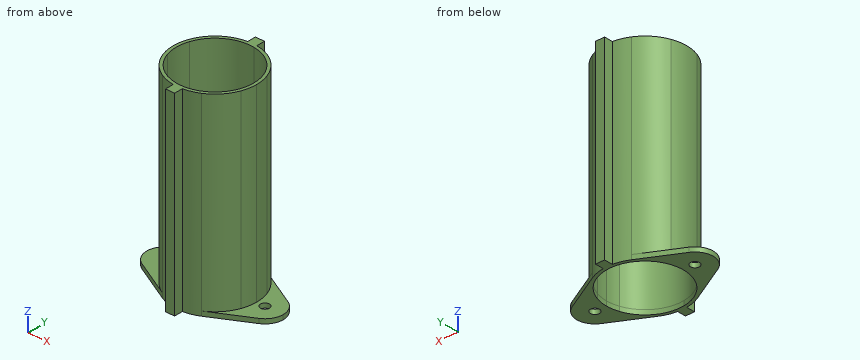
```python
from build123d import *
from build123d import SkipClean  # not in build123d's __all__

# Parameters (mm, degrees)
F0_R     = 3
F1_DEPTH = 3
F2_DEPTH = 125


# Not quite as in the source:
# - a feature names something its author has since deleted; it is built from what else it names


with BuildPart() as f1:
    # F0 (on Top) → F1 (new body)
    with BuildSketch(Plane.XY):
        with BuildLine():
            ThreePointArc((12.9166666896, 24.2777618744), (20.6949130465, 18.1099578685), (25.7765151515, 9.5823413967))
            ThreePointArc((25.7765151515, 9.5823413967), (32.0589540907, 11.9630444535), (38.6363637791, 10.5939323837))
            Line((38.6363637791, 10.5939323837), (12.9166666896, 24.2777618744))
        make_face()
        with BuildLine():
            ThreePointArc((25.7765151515, 9.5823413967), (27.0656993875, 4.8680506023), (27.5, 0))
            ThreePointArc((27.5, 0), (27.0656993875, -4.8680506023), (25.7765151515, -9.5823413967))
            ThreePointArc((25.7765151515, -9.5823413967), (32.0589541175, -11.9630444556), (38.6363638266, -10.5939323584))
            ThreePointArc((38.6363638266, -10.5939323584), (43.2867965353, -6.1791437142), (45, 0))
            ThreePointArc((45, 0), (43.2867965215, 6.1791437372), (38.6363637791, 10.5939323837))
            ThreePointArc((38.6363637791, 10.5939323837), (32.0589540907, 11.9630444535), (25.7765151515, 9.5823413967))
        make_face()
        with Locations((33, 0)):
            Circle(F0_R, mode=Mode.SUBTRACT)
        with BuildLine():
            ThreePointArc((25.7765151515, -9.5823413967), (27.0656993875, -4.8680506023), (27.5, 0))
            ThreePointArc((27.5, 0), (27.0656993875, 4.8680506023), (25.7765151515, 9.5823413967))
            ThreePointArc((25.7765151515, 9.5823413967), (24.9405426226, 8.8907337595), (24.1704545455, 8.1264461523))
            ThreePointArc((24.1704545455, 8.1264461523), (25.1654186425, 4.117244776), (25.5, 0))
            ThreePointArc((25.5, 0), (25.1654186425, -4.117244776), (24.1704545455, -8.1264461523))
            ThreePointArc((24.1704545455, -8.1264461523), (24.9405426226, -8.8907337595), (25.7765151515, -9.5823413967))
        make_face()
        with BuildLine():
            ThreePointArc((-3, 27.3358738657), (0, 27.5), (3, 27.3358738657))
            Line((3, 27.3358738657), (3, 33))
            Line((3, 33), (-3, 33))
            Line((-3, 33), (-3, 27.3358738657))
        make_face()
        with BuildLine():
            ThreePointArc((38.6363638266, -10.5939323584), (32.0589541175, -11.9630444556), (25.7765151515, -9.5823413967))
            ThreePointArc((25.7765151515, -9.5823413967), (20.6949131964, -18.1099576972), (12.9166670915, -24.2777616606))
            Line((12.9166670915, -24.2777616606), (38.6363638266, -10.5939323584))
        make_face()
        with BuildLine():
            ThreePointArc((-25.7765151515, 9.5823413967), (-20.6949129227, 18.1099580099), (-12.9166663578, 24.2777620509))
            Line((-12.9166663578, 24.2777620509), (-38.636363452, 10.5939325577))
            ThreePointArc((-38.636363452, 10.5939325577), (-32.058953906, 11.963044439), (-25.7765151515, 9.5823413967))
        make_face()
        with BuildLine():
            ThreePointArc((-25.7765151515, -9.5823413967), (-27.5, 0), (-25.7765151515, 9.5823413967))
            ThreePointArc((-25.7765151515, 9.5823413967), (-32.058953906, 11.963044439), (-38.636363452, 10.5939325577))
            ThreePointArc((-38.636363452, 10.5939325577), (-45, 1.496e-07), (-38.6363637162, -10.5939324171))
            ThreePointArc((-38.6363637162, -10.5939324171), (-32.0589540552, -11.9630444507), (-25.7765151515, -9.5823413967))
        make_face()
        with Locations((-33, 0)):
            Circle(F0_R, mode=Mode.SUBTRACT)
        with BuildLine():
            ThreePointArc((-24.1704545455, -8.1264461523), (-25.5, 0), (-24.1704545455, 8.1264461523))
            ThreePointArc((-24.1704545455, 8.1264461523), (-24.9405426226, 8.8907337595), (-25.7765151515, 9.5823413967))
            ThreePointArc((-25.7765151515, 9.5823413967), (-27.5, 0), (-25.7765151515, -9.5823413967))
            ThreePointArc((-25.7765151515, -9.5823413967), (-24.9405426226, -8.8907337595), (-24.1704545455, -8.1264461523))
        make_face()
        with BuildLine():
            Line((-38.6363637162, -10.5939324171), (-12.9166665881, -24.2777619284))
            ThreePointArc((-12.9166665881, -24.2777619284), (-20.6949130086, -18.1099579118), (-25.7765151515, -9.5823413967))
            ThreePointArc((-25.7765151515, -9.5823413967), (-32.0589540552, -11.9630444507), (-38.6363637162, -10.5939324171))
        make_face()
        with BuildLine():
            Line((3, 25.3229145242), (3, 27.3358738657))
            ThreePointArc((3, 27.3358738657), (0, 27.5), (-3, 27.3358738657))
            Line((-3, 27.3358738657), (-3, 25.3229145242))
            ThreePointArc((-3, 25.3229145242), (0, 25.5), (3, 25.3229145242))
        make_face()
        with BuildLine():
            ThreePointArc((24.1704545455, 8.1264461523), (24.9405426226, 8.8907337595), (25.7765151515, 9.5823413967))
            ThreePointArc((25.7765151515, 9.5823413967), (20.6949130465, 18.1099578685), (12.9166666896, 24.2777618744))
            ThreePointArc((12.9166666896, 24.2777618744), (8.1038930067, 26.2788302277), (3, 27.3358738657))
            Line((3, 27.3358738657), (3, 25.3229145242))
            ThreePointArc((3, 25.3229145242), (16.0775629735, 19.7929777657), (24.1704545455, 8.1264461523))
        make_face()
        with BuildLine():
            Line((-3, 25.3229145242), (-3, 27.3358738657))
            ThreePointArc((-3, 27.3358738657), (-8.1038928272, 26.2788302831), (-12.9166663578, 24.2777620509))
            ThreePointArc((-12.9166663578, 24.2777620509), (-20.6949129227, 18.1099580099), (-25.7765151515, 9.5823413967))
            ThreePointArc((-25.7765151515, 9.5823413967), (-24.9405426226, 8.8907337595), (-24.1704545455, 8.1264461523))
            ThreePointArc((-24.1704545455, 8.1264461523), (-16.0775629735, 19.7929777657), (-3, 25.3229145242))
        make_face()
        with BuildLine():
            ThreePointArc((-3, -27.3358738657), (0, -27.5), (3, -27.3358738657))
            Line((3, -27.3358738657), (3, -25.3229145242))
            ThreePointArc((3, -25.3229145242), (0, -25.5), (-3, -25.3229145242))
            Line((-3, -25.3229145242), (-3, -27.3358738657))
        make_face()
        with BuildLine():
            Line((3, -33), (3, -27.3358738657))
            ThreePointArc((3, -27.3358738657), (0, -27.5), (-3, -27.3358738657))
            Line((-3, -27.3358738657), (-3, -33))
            Line((-3, -33), (3, -33))
        make_face()
        with BuildLine():
            ThreePointArc((12.9166670915, -24.2777616606), (20.6949131964, -18.1099576972), (25.7765151515, -9.5823413967))
            ThreePointArc((25.7765151515, -9.5823413967), (24.9405426226, -8.8907337595), (24.1704545455, -8.1264461523))
            ThreePointArc((24.1704545455, -8.1264461523), (16.0775629735, -19.7929777657), (3, -25.3229145242))
            Line((3, -25.3229145242), (3, -27.3358738657))
            ThreePointArc((3, -27.3358738657), (8.1038932243, -26.2788301606), (12.9166670915, -24.2777616606))
        make_face()
        with BuildLine():
            ThreePointArc((-12.9166665881, -24.2777619284), (-8.1038929518, -26.2788302446), (-3, -27.3358738657))
            Line((-3, -27.3358738657), (-3, -25.3229145242))
            ThreePointArc((-3, -25.3229145242), (-16.0775629735, -19.7929777657), (-24.1704545455, -8.1264461523))
            ThreePointArc((-24.1704545455, -8.1264461523), (-24.9405426226, -8.8907337595), (-25.7765151515, -9.5823413967))
            ThreePointArc((-25.7765151515, -9.5823413967), (-20.6949130086, -18.1099579118), (-12.9166665881, -24.2777619284))
        make_face()
    extrude(amount=-F1_DEPTH)

    # F0 (on Top) → F2 (join)
    with BuildSketch(Plane.XY):
        with BuildLine():
            Line((-3, 25.3229145242), (-3, 27.3358738657))
            ThreePointArc((-3, 27.3358738657), (-8.1038928272, 26.2788302831), (-12.9166663578, 24.2777620509))
            ThreePointArc((-12.9166663578, 24.2777620509), (-20.6949129227, 18.1099580099), (-25.7765151515, 9.5823413967))
            ThreePointArc((-25.7765151515, 9.5823413967), (-24.9405426226, 8.8907337595), (-24.1704545455, 8.1264461523))
            ThreePointArc((-24.1704545455, 8.1264461523), (-16.0775629735, 19.7929777657), (-3, 25.3229145242))
        make_face()
        with BuildLine():
            ThreePointArc((-3, 27.3358738657), (0, 27.5), (3, 27.3358738657))
            Line((3, 27.3358738657), (3, 33))
            Line((3, 33), (-3, 33))
            Line((-3, 33), (-3, 27.3358738657))
        make_face()
        with BuildLine():
            Line((3, 25.3229145242), (3, 27.3358738657))
            ThreePointArc((3, 27.3358738657), (0, 27.5), (-3, 27.3358738657))
            Line((-3, 27.3358738657), (-3, 25.3229145242))
            ThreePointArc((-3, 25.3229145242), (0, 25.5), (3, 25.3229145242))
        make_face()
        with BuildLine():
            ThreePointArc((24.1704545455, 8.1264461523), (24.9405426226, 8.8907337595), (25.7765151515, 9.5823413967))
            ThreePointArc((25.7765151515, 9.5823413967), (20.6949130465, 18.1099578685), (12.9166666896, 24.2777618744))
            ThreePointArc((12.9166666896, 24.2777618744), (8.1038930067, 26.2788302277), (3, 27.3358738657))
            Line((3, 27.3358738657), (3, 25.3229145242))
            ThreePointArc((3, 25.3229145242), (16.0775629735, 19.7929777657), (24.1704545455, 8.1264461523))
        make_face()
        with BuildLine():
            Line((3, -33), (3, -27.3358738657))
            ThreePointArc((3, -27.3358738657), (0, -27.5), (-3, -27.3358738657))
            Line((-3, -27.3358738657), (-3, -33))
            Line((-3, -33), (3, -33))
        make_face()
        with BuildLine():
            ThreePointArc((-24.1704545455, -8.1264461523), (-25.5, 0), (-24.1704545455, 8.1264461523))
            ThreePointArc((-24.1704545455, 8.1264461523), (-24.9405426226, 8.8907337595), (-25.7765151515, 9.5823413967))
            ThreePointArc((-25.7765151515, 9.5823413967), (-27.5, 0), (-25.7765151515, -9.5823413967))
            ThreePointArc((-25.7765151515, -9.5823413967), (-24.9405426226, -8.8907337595), (-24.1704545455, -8.1264461523))
        make_face()
        with BuildLine():
            ThreePointArc((25.7765151515, -9.5823413967), (27.0656993875, -4.8680506023), (27.5, 0))
            ThreePointArc((27.5, 0), (27.0656993875, 4.8680506023), (25.7765151515, 9.5823413967))
            ThreePointArc((25.7765151515, 9.5823413967), (24.9405426226, 8.8907337595), (24.1704545455, 8.1264461523))
            ThreePointArc((24.1704545455, 8.1264461523), (25.1654186425, 4.117244776), (25.5, 0))
            ThreePointArc((25.5, 0), (25.1654186425, -4.117244776), (24.1704545455, -8.1264461523))
            ThreePointArc((24.1704545455, -8.1264461523), (24.9405426226, -8.8907337595), (25.7765151515, -9.5823413967))
        make_face()
        with BuildLine():
            ThreePointArc((-3, -27.3358738657), (0, -27.5), (3, -27.3358738657))
            Line((3, -27.3358738657), (3, -25.3229145242))
            ThreePointArc((3, -25.3229145242), (0, -25.5), (-3, -25.3229145242))
            Line((-3, -25.3229145242), (-3, -27.3358738657))
        make_face()
        with BuildLine():
            ThreePointArc((-12.9166665881, -24.2777619284), (-8.1038929518, -26.2788302446), (-3, -27.3358738657))
            Line((-3, -27.3358738657), (-3, -25.3229145242))
            ThreePointArc((-3, -25.3229145242), (-16.0775629735, -19.7929777657), (-24.1704545455, -8.1264461523))
            ThreePointArc((-24.1704545455, -8.1264461523), (-24.9405426226, -8.8907337595), (-25.7765151515, -9.5823413967))
            ThreePointArc((-25.7765151515, -9.5823413967), (-20.6949130086, -18.1099579118), (-12.9166665881, -24.2777619284))
        make_face()
        with BuildLine():
            ThreePointArc((12.9166670915, -24.2777616606), (20.6949131964, -18.1099576972), (25.7765151515, -9.5823413967))
            ThreePointArc((25.7765151515, -9.5823413967), (24.9405426226, -8.8907337595), (24.1704545455, -8.1264461523))
            ThreePointArc((24.1704545455, -8.1264461523), (16.0775629735, -19.7929777657), (3, -25.3229145242))
            Line((3, -25.3229145242), (3, -27.3358738657))
            ThreePointArc((3, -27.3358738657), (8.1038932243, -26.2788301606), (12.9166670915, -24.2777616606))
        make_face()
    with SkipClean():  # cleaning this boolean's faces spoils the solid; the shape is the same uncleaned
        extrude(amount=F2_DEPTH)


solid = f1.part
```
The model under review builds one solid part; all positions refer to its coordinate system, in mm. Give positions to 0.01 mm unless a question says otherwise; leave off trailing zeros. Loops run counter-clockwise (first coordinate to the right, second up) from the corner with the lowest first, then second, coordinate; pieces in that order, holes last. Notation, with made-up numbers: (-1, 85.25) -> (28, 85.25) arc R30 cw to (28, 114.25) -> close; hole circle Ø9 at (-1.75, 20). An arc over 180 degrees is marked (long way). Use CSV: the item, a comma, the result in double quotes.
1. Consider section C-C, the plane x = 33. Write out the cut boundary in (y, z).
Result:
outline,"(-13.59, -3) -> (-3, -3) -> (-3, 0) -> (-13.59, 0) -> close; (3, -3) -> (13.59, -3) -> (13.59, 0) -> (3, 0) -> close"
2. To check wall thickness, follow probe 1 along Z at (x, y) = (-29, 15.5); probe 2 along Y at (x, z) = (17.5, 110.5); probe 3 along Y at (x, z) = (-5, 33) (3 decimals). State the ranges of each line that lie inside material, in increasing order. Write a range as from..to.
Result:
probe 1,"z = -3..0"
probe 2,"y = -21.21..-18.55, 18.55..21.21"
probe 3,"y = -27.042..-25.005, 25.005..27.042"
3. Consider section B-B, the plane y = 16.5. Write out the cut boundary in (x, z), then the cut area to 3 significant figures.
Result:
outline,"(-27.54, -3) -> (-19.44, -3) -> (-19.44, 125) -> (-22, 125) -> (-22, 0) -> (-27.54, 0) -> close; (19.44, -3) -> (27.54, -3) -> (27.54, 0) -> (22, 0) -> (22, 125) -> (19.44, 125) -> close"
area,"688 mm²"
4. Consider section A-A, the plane z = 95. Write out the cut boundary in (x, y), then the cut area to 3 significant figures.
Result:
outline,"(-3, -33) -> (3, -33) -> (3, -27.34) arc R27.5 ccw to (3, 27.34) -> (3, 33) -> (-3, 33) -> (-3, 27.34) arc R27.5 ccw to (-3, -27.34) -> close; hole circle Ø51 at (0, 0)"
area,"400 mm²"
5. For P1, Ø3, axis at y = 13.5, z = 103.5, coming from the -X side; P2, Ø1.7, axis at y = -30, z = 56, coming from the -X side; P3, Ø5, axis at y = -3, z = 74.5, coming from the +X side; P4, Ø6, axis at x = -33, y = -19.5, coming from the -Z side, all flat-tipped, find the tip position at first contact; note any pin that passes through.
Result:
P1,"stops at x = -24.74"
P2,"stops at x = -3"
P3,"stops at x = 27.5"
P4,"passes through"
6. Consider section D-D, the plane x = -20. Write out the cut boundary in (y, z).
Result:
outline,"(-20.51, -3) -> (-15.82, -3) -> (-15.82, 125) -> (-18.87, 125) -> (-18.87, 0) -> (-20.51, 0) -> close; (15.82, -3) -> (20.51, -3) -> (20.51, 0) -> (18.87, 0) -> (18.87, 125) -> (15.82, 125) -> close"
